Geometry: final body of the model. Coordinates: model frame, mm. A direction names the side the tool comes from. Coordinates: 2 decimals unless noted, no trailing zeros. Loops run counter-clockwise (first coordinate to the right, second up) from the corner with the lowest first, then second, coordinate; pieces in that order, holes last. Notation, with made-up numbers: (-15, 57.25) -> (-8, 57.25) arc R16 cw to (-8, 70.25) -> close; hole circle Ø10 at (-15.5, 33). An arc over 180 degrees is marked (long way). One line per item, written item: value. Start each with the question number.
Item 1: Section query A-A on z = 0. Return loops of the section in (x, y) (3 decimals), then the cut area to 3 significant figures.
Item 2: Section query C-C on z = -161. Return loops of the section in (x, y) (3 decimals), then the cut area to 3 significant figures.
Item 3: Contact query for flat-ended pins moving along their axis: pin 1 Ø12.5 at (y, z) = (48.5, -209.5) entering from +X; pin 2 Ø5 at (y, z) = (79.5, 184.5) entering from +X. Output: stop coordinate, or through.
Item 4: Section query D-D on z = -228. Return loops of the section in (x, y) (3 decimals), then the cut area to 3 significant figures.
Item 5: Ray query, probe 1 along Y at (x, z) = (0.85, -298.45); probe 2 along Y at (x, z) = (20.5, 171) (3 decimals); probe 3 along Y at (x, z) = (0.85, 0). Return the intervals inside material, ascending. Write a range as from..to.
Item 6: Set-up query: faces 4 (the flat face through (1.6, 51, -162)), 5 (the flat face through (0.81, 53.49, -241.67)). Return all of +Z, -Z, +X, -X, +Y, -Y with unobstructed straight access to the full face (end or side cutting, diameter ignored); none if empty.
Item 7: Section query B-B on x = 12.75. Return loops of the section in (y, z) (3 decimals).
Item 8: Mould query, pull axis Z, two halves, no side actions, for faces 1 (the flat face through (1, 51, 304.8)), 2 (the flat face through (1.6, 50, -299)), 3 (the flat face through (0.81, 48.11, 172.14)). Classes: +Z half, -Z half, draft (parallel to the pull), parting line (faces both ways), or undercut.
from build123d import *

# Parameters (mm, degrees)
SKETCH1_W           = 1.6002
SKETCH1_H           = 101.6
BOSS_EXTRUDE1_DEPTH = 304.8
BOSS_EXTRUDE2_DEPTH = 304.8
SKETCH3_R           = 19.05
CUT_EXTRUDE1_DEPTH  = 323.289869527
SKETCH4_R           = 3.175
CUT_EXTRUDE2_DEPTH  = 323.289869527
SKETCH5_R           = 3.175
CUT_EXTRUDE3_DEPTH  = 323.289869527


with BuildPart() as part:
    # Sketch1 → Boss-Extrude1 (new, symmetric)
    with BuildSketch(Plane.XY):
        with Locations((0.8001, 50.8)):
            Rectangle(SKETCH1_W, SKETCH1_H)
    extrude(amount=BOSS_EXTRUDE1_DEPTH, both=True)

    # Sketch2 → Boss-Extrude2 (add, symmetric)
    with BuildSketch(Plane.XY):
        with BuildLine():
            Line((27.0002, 101.6), (1.6002, 101.6))
            Line((1.6002, 101.6), (1.6002, 76.2))
            ThreePointArc((1.6002, 76.2), (3.84526403, 77.12993597), (4.7752, 79.375))
            Line((4.7752, 79.375), (4.7752, 95.25))
            ThreePointArc((4.7752, 95.25), (5.70513597, 97.49506403), (7.9502, 98.425))
            Line((7.9502, 98.425), (23.8252, 98.425))
            ThreePointArc((23.8252, 98.425), (26.07026403, 99.35493597), (27.0002, 101.6))
        make_face()
        with BuildLine():
            Line((7.9502, 3.175), (23.8252, 3.175))
            ThreePointArc((23.8252, 3.175), (26.07026403, 2.24506403), (27.0002, 0))
            Line((27.0002, 0), (1.6002, 0))
            Line((1.6002, 0), (1.6002, 25.4))
            ThreePointArc((1.6002, 25.4), (3.84526403, 24.47006403), (4.7752, 22.225))
            Line((4.7752, 22.225), (4.7752, 6.35))
            ThreePointArc((4.7752, 6.35), (5.70513597, 4.10493597), (7.9502, 3.175))
        make_face()
    extrude(amount=BOSS_EXTRUDE2_DEPTH, both=True)

    # Sketch3 → Cut-Extrude1 (cut, through all)
    with BuildSketch(Plane(origin=(1.6002, 0, 0), x_dir=(0, 0, -1), z_dir=(1, 0, 0))):
        with Locations((0, 50.8)):
            Circle(SKETCH3_R)
        with BuildLine():
            Line((-292.1, 73.025), (-292.1, 28.575))
            ThreePointArc((-292.1, 28.575), (-290.227720313, 25.679564837), (-286.819026907, 26.198973416))
            Line((-286.819026907, 26.198973416), (-236.669107137, 70.648973416))
            ThreePointArc((-236.669107137, 70.648973416), (-235.806536024, 74.151219471), (-238.77508023, 76.2))
            Line((-238.77508023, 76.2), (-288.925, 76.2))
            ThreePointArc((-288.925, 76.2), (-291.17006403, 75.27006403), (-292.1, 73.025))
        make_face()
        with BuildLine():
            Line((-264.991586436, 25.4), (-214.841666667, 25.4))
            ThreePointArc((-214.841666667, 25.4), (-212.596602636, 26.32993597), (-211.666666667, 28.575))
            Line((-211.666666667, 28.575), (-211.666666667, 73.025))
            ThreePointArc((-211.666666667, 73.025), (-213.538946354, 75.920435163), (-216.94763976, 75.401026584))
            Line((-216.94763976, 75.401026584), (-267.09755953, 30.951026584))
            ThreePointArc((-267.09755953, 30.951026584), (-267.960130642, 27.448780529), (-264.991586436, 25.4))
        make_face()
        with BuildLine():
            Line((-202.141666667, 73.025), (-202.141666667, 28.575))
            ThreePointArc((-202.141666667, 28.575), (-200.26938698, 25.679564837), (-196.860693573, 26.198973416))
            Line((-196.860693573, 26.198973416), (-146.710773804, 70.648973416))
            ThreePointArc((-146.710773804, 70.648973416), (-145.848202691, 74.151219471), (-148.816746897, 76.2))
            Line((-148.816746897, 76.2), (-198.966666667, 76.2))
            ThreePointArc((-198.966666667, 76.2), (-201.211730697, 75.27006403), (-202.141666667, 73.025))
        make_face()
        with BuildLine():
            Line((-126.989306427, 75.401026584), (-177.139226196, 30.951026584))
            ThreePointArc((-177.139226196, 30.951026584), (-178.001797309, 27.448780529), (-175.033253103, 25.4))
            Line((-175.033253103, 25.4), (-124.883333333, 25.4))
            ThreePointArc((-124.883333333, 25.4), (-122.638269303, 26.32993597), (-121.708333333, 28.575))
            Line((-121.708333333, 28.575), (-121.708333333, 73.025))
            ThreePointArc((-121.708333333, 73.025), (-123.58061302, 75.920435163), (-126.989306427, 75.401026584))
        make_face()
        with BuildLine():
            Line((-112.183333333, 73.025), (-112.183333333, 28.575))
            ThreePointArc((-112.183333333, 28.575), (-110.311053646, 25.679564837), (-106.90236024, 26.198973416))
            Line((-106.90236024, 26.198973416), (-56.75244047, 70.648973416))
            ThreePointArc((-56.75244047, 70.648973416), (-55.889869358, 74.151219471), (-58.858413564, 76.2))
            Line((-58.858413564, 76.2), (-109.008333333, 76.2))
            ThreePointArc((-109.008333333, 76.2), (-111.253397364, 75.27006403), (-112.183333333, 73.025))
        make_face()
        with BuildLine():
            Line((-37.030973093, 75.401026584), (-87.180892863, 30.951026584))
            ThreePointArc((-87.180892863, 30.951026584), (-88.043463976, 27.448780529), (-85.07491977, 25.4))
            Line((-85.07491977, 25.4), (-34.925, 25.4))
            ThreePointArc((-34.925, 25.4), (-32.67993597, 26.32993597), (-31.75, 28.575))
            Line((-31.75, 28.575), (-31.75, 73.025))
            ThreePointArc((-31.75, 73.025), (-33.622279687, 75.920435163), (-37.030973093, 75.401026584))
        make_face()
        with BuildLine():
            Line((85.07491977, 25.4), (34.925, 25.4))
            ThreePointArc((34.925, 25.4), (32.67993597, 26.32993597), (31.75, 28.575))
            Line((31.75, 28.575), (31.75, 73.025))
            ThreePointArc((31.75, 73.025), (33.622279687, 75.920435163), (37.030973093, 75.401026584))
            Line((37.030973093, 75.401026584), (87.180892863, 30.951026584))
            ThreePointArc((87.180892863, 30.951026584), (88.043463976, 27.448780529), (85.07491977, 25.4))
        make_face()
        with BuildLine():
            Line((56.75244047, 70.648973416), (106.90236024, 26.198973416))
            ThreePointArc((106.90236024, 26.198973416), (110.311053646, 25.679564837), (112.183333333, 28.575))
            Line((112.183333333, 28.575), (112.183333333, 73.025))
            ThreePointArc((112.183333333, 73.025), (111.253397364, 75.27006403), (109.008333333, 76.2))
            Line((109.008333333, 76.2), (58.858413564, 76.2))
            ThreePointArc((58.858413564, 76.2), (55.889869358, 74.151219471), (56.75244047, 70.648973416))
        make_face()
        with BuildLine():
            Line((175.033253103, 25.4), (124.883333333, 25.4))
            ThreePointArc((124.883333333, 25.4), (122.638269303, 26.32993597), (121.708333333, 28.575))
            Line((121.708333333, 28.575), (121.708333333, 73.025))
            ThreePointArc((121.708333333, 73.025), (123.58061302, 75.920435163), (126.989306427, 75.401026584))
            Line((126.989306427, 75.401026584), (177.139226196, 30.951026584))
            ThreePointArc((177.139226196, 30.951026584), (178.001797309, 27.448780529), (175.033253103, 25.4))
        make_face()
        with BuildLine():
            Line((146.710773804, 70.648973416), (196.860693573, 26.198973416))
            ThreePointArc((196.860693573, 26.198973416), (200.26938698, 25.679564837), (202.141666667, 28.575))
            Line((202.141666667, 28.575), (202.141666667, 73.025))
            ThreePointArc((202.141666667, 73.025), (201.211730697, 75.27006403), (198.966666667, 76.2))
            Line((198.966666667, 76.2), (148.816746897, 76.2))
            ThreePointArc((148.816746897, 76.2), (145.848202691, 74.151219471), (146.710773804, 70.648973416))
        make_face()
        with BuildLine():
            Line((216.94763976, 75.401026584), (267.09755953, 30.951026584))
            ThreePointArc((267.09755953, 30.951026584), (267.960130642, 27.448780529), (264.991586436, 25.4))
            Line((264.991586436, 25.4), (214.841666667, 25.4))
            ThreePointArc((214.841666667, 25.4), (212.596602636, 26.32993597), (211.666666667, 28.575))
            Line((211.666666667, 28.575), (211.666666667, 73.025))
            ThreePointArc((211.666666667, 73.025), (213.538946354, 75.920435163), (216.94763976, 75.401026584))
        make_face()
        with BuildLine():
            Line((236.669107137, 70.648973416), (286.819026907, 26.198973416))
            ThreePointArc((286.819026907, 26.198973416), (290.227720313, 25.679564837), (292.1, 28.575))
            Line((292.1, 28.575), (292.1, 73.025))
            ThreePointArc((292.1, 73.025), (291.17006403, 75.27006403), (288.925, 76.2))
            Line((288.925, 76.2), (238.77508023, 76.2))
            ThreePointArc((238.77508023, 76.2), (235.806536024, 74.151219471), (236.669107137, 70.648973416))
        make_face()
    extrude(amount=-CUT_EXTRUDE1_DEPTH, mode=Mode.SUBTRACT)

    # Sketch4 → Cut-Extrude2 (cut, through all)
    with BuildSketch(Plane(origin=(1.6002, 0, 0), x_dir=(0, 0, -1), z_dir=(1, 0, 0))):
        with Locations((-22.225, 73.025)):
            Circle(SKETCH4_R)
        with Locations((22.225, 73.025)):
            Circle(SKETCH4_R)
        with Locations((22.225, 28.575)):
            Circle(SKETCH4_R)
        with Locations((-22.225, 28.575)):
            Circle(SKETCH4_R)
    extrude(amount=-CUT_EXTRUDE2_DEPTH, mode=Mode.SUBTRACT)

    # Sketch5 → Cut-Extrude3 (cut, through all)
    with BuildSketch(Plane(origin=(1.6002, 0, 0), x_dir=(0, 0, -1), z_dir=(1, 0, 0))):
        with Locations((-298.45, 66.675)):
            Circle(SKETCH5_R)
        with Locations((-298.45, 34.925)):
            Circle(SKETCH5_R)
        with Locations(Location((298.45, 34.925, 0), (0, 0, 180))):
            Circle(SKETCH5_R)
        with Locations(Location((298.45, 66.675, 0), (0, 0, 180))):
            Circle(SKETCH5_R)
    extrude(amount=-CUT_EXTRUDE3_DEPTH, mode=Mode.SUBTRACT)


solid = part.part
Reply:
1. outline: (0, 0) -> (27, 0) arc R3.175 ccw to (23.825, 3.175) -> (7.95, 3.175) arc R3.175 cw to (4.775, 6.35) -> (4.775, 22.225) arc R3.175 ccw to (1.6, 25.4) -> (1.6, 31.75) -> (0, 31.75) -> close; (0, 69.85) -> (1.6, 69.85) -> (1.6, 76.2) arc R3.175 ccw to (4.775, 79.375) -> (4.775, 95.25) arc R3.175 cw to (7.95, 98.425) -> (23.825, 98.425) arc R3.175 ccw to (27, 101.6) -> (0, 101.6) -> close
1. area: 400 mm²
2. outline: (0, 0) -> (27, 0) arc R3.175 ccw to (23.825, 3.175) -> (7.95, 3.175) arc R3.175 cw to (4.775, 6.35) -> (4.775, 22.225) arc R3.175 ccw to (1.6, 25.4) -> (0, 25.4) -> close; (0, 45.256) -> (1.6, 45.256) -> (1.6, 57.984) -> (0, 57.984) -> close; (0, 76.2) -> (1.6, 76.2) arc R3.175 ccw to (4.775, 79.375) -> (4.775, 95.25) arc R3.175 cw to (7.95, 98.425) -> (23.825, 98.425) arc R3.175 ccw to (27, 101.6) -> (0, 101.6) -> close
2. area: 400 mm²
3. pin 1: stops at x = 1.6
3. pin 2: stops at x = 4.78
4. outline: (0, 0) -> (27, 0) arc R3.175 ccw to (23.825, 3.175) -> (7.95, 3.175) arc R3.175 cw to (4.775, 6.35) -> (4.775, 22.225) arc R3.175 ccw to (1.6, 25.4) -> (0, 25.4) -> close; (0, 65.605) -> (1.6, 65.605) -> (1.6, 76.2) arc R3.175 ccw to (4.775, 79.375) -> (4.775, 95.25) arc R3.175 cw to (7.95, 98.425) -> (23.825, 98.425) arc R3.175 ccw to (27, 101.6) -> (0, 101.6) -> close
4. area: 396 mm²
5. probe 1: y = 0..31.75, 38.1..63.5, 69.85..101.6
5. probe 2: y = 0..3.175, 98.425..101.6
5. probe 3: y = 0..31.75, 69.85..101.6
6. face 4: +Z, -Z, +X
6. face 5: +X, -X
7. outline: (0, -304.8) -> (3.175, -304.8) -> (3.175, 304.8) -> (0, 304.8) -> close; (98.425, -304.8) -> (101.6, -304.8) -> (101.6, 304.8) -> (98.425, 304.8) -> close
8. face 1: +Z half
8. face 2: draft
8. face 3: undercut
